Work out the finished part from the listing and answer in its coordinate system (mm). A direction names the side the tool comes from. Round coordinates to 2 decimals unless told otherwise and drop trailing zeros. Write each loop counter-clockwise with the first axis right and the second up, starting at its lowest first coordinate (ties: lowest second). Pieces come first, ordered by that corner, then holes. Notation, with made-up numbers: (18, 50) -> (32, 50) arc R4 cw to (32, 57) -> close; hole circle Ø6 at (3.25, 55). An arc over 180 degrees is marked (long way). One line per question, with ' | ' between items. Start each with the question number.
```python
from build123d import *

# Parameters (mm, degrees)
EXTRUDE_1_DEPTH     = 1.04
CUT_EXTRUDE_1_DEPTH = 1.04
SKETCH_4_W          = 8.4
SKETCH_4_H          = 3
EXTRUDE_2_DEPTH     = 2.4
CHAMFER_1_SIZE      = 1.2
CHAMFER_1_SIZE_2    = 2.4


with BuildPart() as part:
    # Эскиз1 → Бобышка-Вытянуть1 (new body)
    with BuildSketch(Plane.XY):
        with BuildLine():
            Line((-4.6, 0), (-4.6, 6.174949393))
            ThreePointArc((-4.6, 6.174949393), (-6.88149693, 3.454706934), (-7.7, 0))
            Line((-7.7, 0), (-7.7, -20.6))
            Line((-7.7, -20.6), (7.7, -20.6))
            Line((7.7, -20.6), (7.7, 0))
            ThreePointArc((7.7, 0), (6.88149693, 3.454706934), (4.6, 6.174949393))
            Line((4.6, 6.174949393), (4.6, 0))
            ThreePointArc((4.6, 0), (0, -4.6), (-4.6, 0))
        make_face()
    extrude(amount=EXTRUDE_1_DEPTH)

    # Эскиз3 → Вырез-Вытянуть1 (cut)
    with BuildSketch(Plane.XY.offset(1.04)):
        with BuildLine():
            Line((-7.7, -20.6), (-4.2, -20.6))
            Line((-4.2, -20.6), (-4.2, -15.2))
            ThreePointArc((-4.2, -15.2), (-5.1372583, -12.9372583), (-7.4, -12))
            Line((-7.4, -12), (-7.7, -12))
            Line((-7.7, -12), (-7.7, -20.6))
        make_face()
        with BuildLine():
            Line((4.2, -20.6), (4.2, -15.2))
            ThreePointArc((4.2, -15.2), (5.1372583, -12.9372583), (7.4, -12))
            Line((7.4, -12), (7.7, -12))
            Line((7.7, -12), (7.7, -20.6))
            Line((7.7, -20.6), (4.2, -20.6))
        make_face()
    extrude(amount=-CUT_EXTRUDE_1_DEPTH, mode=Mode.SUBTRACT)

    # Эскиз4 → Бобышка-Вытянуть2 (add)
    with BuildSketch(Plane.XY.offset(1.04)):
        with Locations((0, -19.1)):
            Rectangle(SKETCH_4_W, SKETCH_4_H)
    extrude(amount=EXTRUDE_2_DEPTH)

    # Фаска1
    # the kernel refuses this chamfer: 2.4, 1.2 mm, written as the material it adds along each edge
    with BuildSketch(Plane(origin=(4.2, -17.6, 1.04), x_dir=(0, 0.9976223042390325, -0.06891834360170876), z_dir=(-1, 0, 0))) as chamfer_1_piece_1_section:
        Polygon((CHAMFER_1_SIZE * 0.997622304239, -CHAMFER_1_SIZE * 0.0689183436017), (-CHAMFER_1_SIZE_2 * 0.0689183436017, -CHAMFER_1_SIZE_2 * 0.997622304239), (0, 0), align=None)
    chamfer_1_piece_1 = extrude(amount=8.4, mode=Mode.PRIVATE)
    chamfer_1_piece_1 = split(chamfer_1_piece_1, bisect_by=Plane(origin=(0, -17.217816218, 3.44), z_dir=(0, 0, -1)), keep=Keep.TOP, mode=Mode.PRIVATE)
    add(chamfer_1_piece_1)


solid = part.part
```
(1) A cutting plane is placed at A-A, the plane x = 0. Determine the outline of the cut face in (y, z), then the cut area to 3 significant figures.
(2) For faces 5 (the flat face through (4.2, -18, 2)), 6 (the flat face through (-4.2, -18, 2)), 7 (the flat face through (0, -7, 1.04)), 8 (the flat face through (4.6, 3.1, 0.5)), determine the directions among +Z, -Z, +X, -X, +Y, -Y from which every point of the face is accessible in a straight line to the end or side of a thin tool.
(3) Given pin 1 Ø4 at (x, y) = (5.5, -14) entering from +Z; pin 2 Ø0.5 at (y, z) = (2, 0.5) entering from -X; pin 3 Ø0.5 at (y, z) = (4, 0.5) entering from +X; pin 4 Ø2 at (x, z) = (4, 1) entering from +Y, each flat-ended and moving along its own axis, determine where each tip first touches the part or whether it passes through.
(4) A cutting plane is placed at D-D, the plane y = -9. Determine the outline of the cut face in (x, z), then the cut area to 3 significant figures.
(5) A cutting plane is placed at C-C, the plane z = 0.3. Determine the outline of the cut face in (x, y), then the cut area to 3 significant figures.
(6) The mould has two halves that part along X. Classify faces 1 (the cylindrical face through (0.1, -4.6, 0.5)), 2 (the flat face through (0, -19, 3.44)), 3 (the flat face through (-4.6, 3, 0.5)), 4 (the cylindrical face through (-5.113, -12.962, 0.527)): +X half, -X half, draft (parallel to the pull), parting line (faces both ways), or undercut.
(7) A cutting plane is placed at B-B, the plane y = 2.5. Determine the outline of the cut face in (x, z).
(8) Consider L1, parallel to Z at x = -1.5, y = -7.5; L2, parallel to X at y = -18.25, z = 1.5; L3, parallel to X at y = -4, z = 0.8. Determine where each line is inside the solid, lowest interval first.
Returned:
1) outline: (-20.6, 0) -> (-4.6, 0) -> (-4.6, 1.04) -> (-16.4, 1.04) -> (-17.6, 3.44) -> (-20.6, 3.44) -> close | area: 25.3 mm2
2) face 5: +Z, -Z, +X, -Y | face 6: +Z, -Z, -X, -Y | face 7: +Z, +X, -X, +Y | face 8: +Z, -Z, +Y
3) pin 1: z = 1.04 | pin 2: x = -7.5 | pin 3: x = 6.73 | pin 4: y = 6.17
4) outline: (-7.7, 0) -> (7.7, 0) -> (7.7, 1.04) -> (-7.7, 1.04) -> close | area: 16.0 mm2
5) outline: (-7.7, -12) -> (-7.4, -12) arc R3.2 cw to (-4.2, -15.2) -> (-4.2, -20.6) -> (4.2, -20.6) -> (4.2, -15.2) arc R3.2 cw to (7.4, -12) -> (7.7, -12) -> (7.7, 0) arc R7.7 ccw to (4.6, 6.17) -> (4.6, 0) arc R4.6 cw to (-4.6, 0) -> (-4.6, 6.17) arc R7.7 ccw to (-7.7, 0) -> close | area: 255 mm2
6) face 1: undercut | face 2: draft | face 3: undercut | face 4: -X half
7) outline: (-7.28, 0) -> (-4.6, 0) -> (-4.6, 1.04) -> (-7.28, 1.04) -> close; (4.6, 0) -> (7.28, 0) -> (7.28, 1.04) -> (4.6, 1.04) -> close
8) L1: 0 to 1.04 | L2: -4.2 to 4.2 | L3: -7.7 to -2.27, 2.27 to 7.7
